Can you work these out from the drawing? Everything is in mm from the part's minimum corner. Coordinates: 2 decimals unless noted, no trailing zeros. Order: outer loops, then holes, each group sorted by start corner. A loop starts at its lowest first (then second) coordinate and runs counter-clockwise, first axis right, second up. Notation, with made-up numbers: (79.25, -33.5) -> (84.25, -33.5) arc R14 cw to (84.25, -24.5) -> close; hole circle Ø7 at (4.5, 20.5). An arc over 180 degrees is marked (long way). Answer in a Markdown table with one row per item.
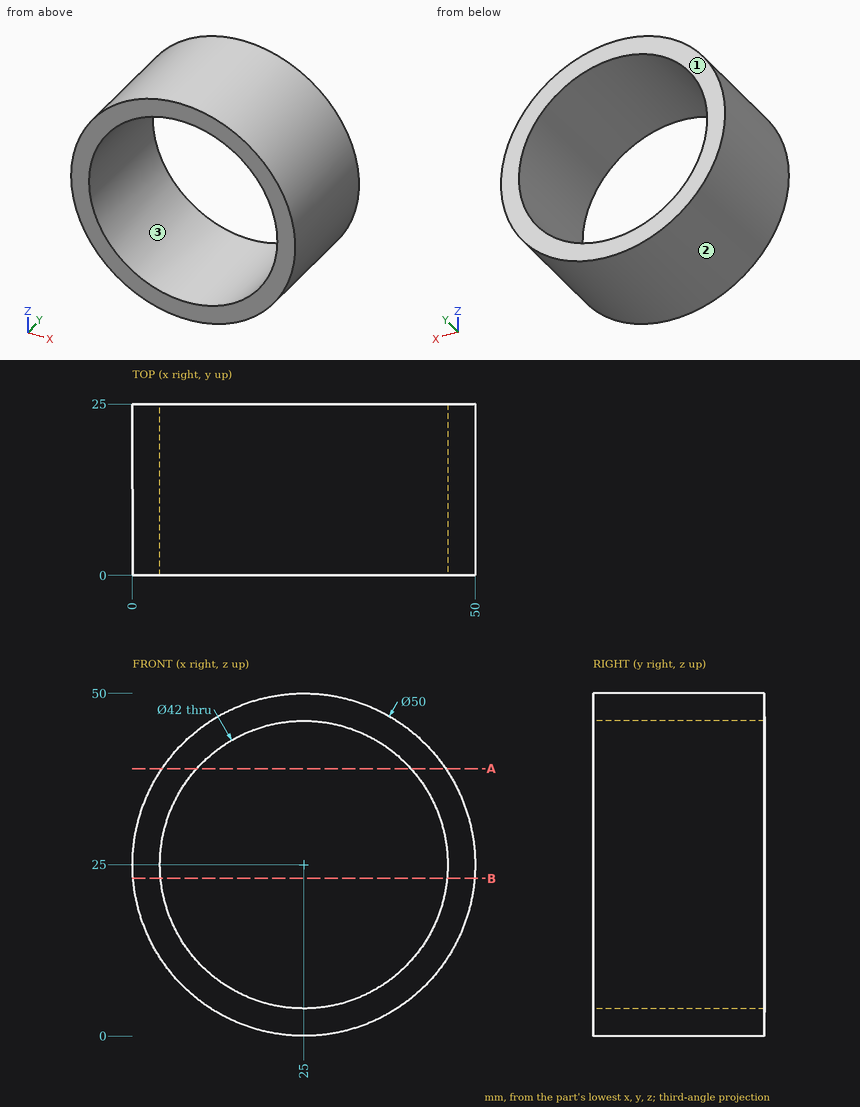
(1) Suppose I cut it at A-A (z = 39). Please give me the cut outline in (x, y).
Response values:
| item | result |
|---|---|
| outline | (4.29, 0) -> (9.35, 0) -> (9.35, 25) -> (4.29, 25) -> close; (40.65, 0) -> (45.71, 0) -> (45.71, 25) -> (40.65, 25) -> close |
(2) I need wall thicknesses on line 1 (X direction, y = 7.5, z = 25); line 2 (X direction, y = 16.25, z = 22.5); line 3 (Z direction, x = 11.5, y = 2.75). Which ranges of each line are inside material? Lowest first, please. Write a range as [from, to].
Response values:
| item | result |
|---|---|
| line 1 | [0, 4], [46, 50] |
| line 2 | [0.13, 4.15], [45.85, 49.87] |
| line 3 | [3.96, 8.91], [41.09, 46.04] |
(3) Suppose I cut it at B-B (z = 23). Please give me the cut outline in (x, y), and give its area (3 significant figures).
Response values:
| item | result |
|---|---|
| outline | (0.08, 0) -> (4.1, 0) -> (4.1, 25) -> (0.08, 25) -> close; (45.9, 0) -> (49.92, 0) -> (49.92, 25) -> (45.9, 25) -> close |
| area | 201 mm2 |
(4) Will these pins go through, and if not, where does the flat tip stop? pin 1 Ø6 at (y, z) = (6, 23.5) entering from -X; pin 2 Ø6 at (x, z) = (17, 38.5) entering from +Y; pin 3 Ø3 at (x, y) = (31.5, 17) entering from +Z; pin 4 Ø1 at (y, z) = (2.5, 13.5) entering from -X.
Response values:
| item | result |
|---|---|
| pin 1 | x = 0 |
| pin 2 | through |
| pin 3 | z = 49.49 |
| pin 4 | x = 2.55 |
(5) We'd pull the mould along Z, two halves only. Please class the marked faces 1, 2 and 3: +Z half, -Z half, draft (parallel to the pull), parting line (faces both ways), or undercut.
Response values:
| item | result |
|---|---|
| face 1 | draft |
| face 2 | parting line |
| face 3 | undercut |
